Geometry check sheet. Reference: drawing and pictorial views, mm from the part's lowest x, y, z. A direction names the side the tool comes from. Coordinates: 2 decimals unless noted, no trailing zeros. Write each loop counter-clockwise with the first axis right and the second up, starting at its lowest first coordinate (ties: lowest second). Pieces come first, ordered by that corner, then holes.
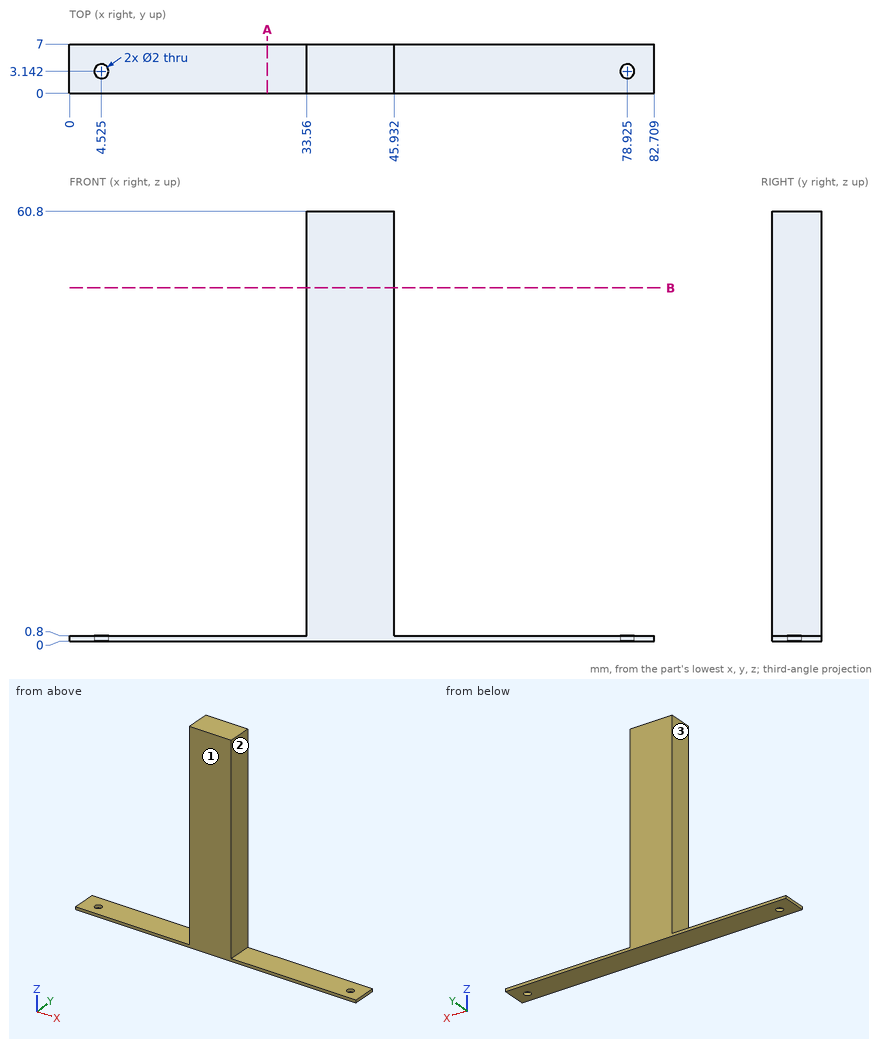
1. Sectioned sample at B-B, the plane z = 50. Record the boundary of the cut face in (x, y), and give its area (3 significant figures).
2. Tool access check on the marked faces 1, 2 and 3. Record the directions out of +Z, -Z, +X, -X, +Y, -Y that give a thin tool (end or side, any length) a straight path to the whole face; none if there is none.
3. Sectioned sample at A-A, the plane x = 28. Record the boundary of the cut face in (y, z).
4. Gauge pin test, flat ends, axial feed: P1, Ø2, axis at y = 4.5, z = 26.5, coming from the +X side; P2, Ø2, axis at x = 11.5, y = 5, coming from the +Z side; P3, Ø3, axis at y = 5.5, z = 30.5, coming from the -X side. Record the tip position at first contact, or that the pin passes through.
5. Material ranges on L1, parallel to Z at x = 16, y = 6.5; L2, parallel to X at y = 4.25, z = 21, recorded low to high.
Outcome:
1. outline: (33.56, 0) - (45.93, 0) - (45.93, 7) - (33.56, 7) - close
1. area: 86.6 mm2
2. face 1: +Z, -Z, +X, -X, -Y
2. face 2: +Z, +X, +Y, -Y
2. face 3: +Z, -X, +Y, -Y
3. outline: (0, 0) - (7, 0) - (7, 0.8) - (0, 0.8) - close
4. P1: stops at x = 45.93
4. P2: stops at z = 0.8
4. P3: stops at x = 33.56
5. L1: z = 0 to 0.8
5. L2: x = 33.56 to 45.93
